The drawing under review shows one solid part. Ordinate dimensions are in mm from its lowest x, y, z. A direction names the side the tool comes from. Round coordinates to 2 decimals unless told otherwise and drop trailing zeros. Write each loop counter-clockwise with the first axis right and the second up, starting at its lowest first coordinate (ties: lowest second). Pieces come first, ordered by that corner, then holes. Notation, with made-up numbers: M 68.25,36.5 L 95.25,36.5 A17 cw 95.25,52.5 Z; hole C 74.25,16.25 d7. An arc over 180 degrees is marked long. Write item = value, one per line. Start each with the question number.
Item 1: Take a section at A-A, the plane y = 13. Give the boundary of the cut face in (x, z).
Item 2: To check wall thickness, follow line 1 along Z through (x, y) = (103.5, 17.75); line 2 along Z through (x, y) = (57.5, 19.75); line 3 along Z through (x, y) = (77, 12.5). State the ranges of each line that lie inside material, in increasing order.
Item 3: Take a section at D-D, the plane x = 87. Give the boundary of the cut face in (y, z), plus the area to 3 significant figures.
Item 4: Take a section at B-B, the plane x = 28. Give the boundary of the cut face in (y, z).
Item 5: For pin 1 Ø3 at (x, y) = (99.5, 6.5) entering from +Z; pin 2 Ø1.2 at (x, z) = (68, 95) entering from -Y; pin 3 Ø10 at (y, z) = (14, 183) entering from +X, all flat-tipped, find the tip position at first contact; note any pin that passes through.
Item 6: Take a section at C-C, the plane z = 54.5. Give the boundary of the cut face in (x, y).
Item 7: Tool access review of the marked faces 1, 2 and 3: name each direction out of +Z, -Z, +X, -X, +Y, -Y from which nothing blocks a thin tool from reaching the whole face with its end or side.
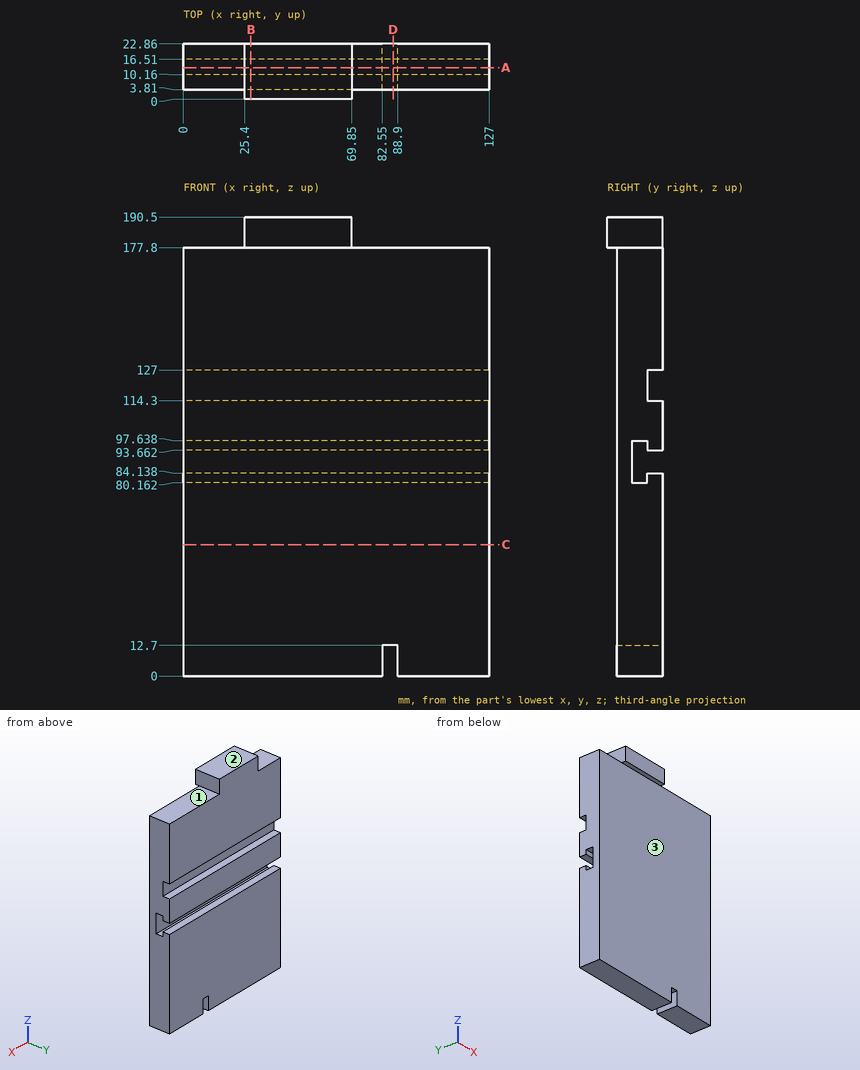
Response values:
q1.outline = M 0,0 L 82.55,0 L 82.55,12.7 L 88.9,12.7 L 88.9,0 L 127,0 L 127,80.16 L 0,80.16 Z; M 0,97.64 L 127,97.64 L 127,177.8 L 69.85,177.8 L 69.85,190.5 L 25.4,190.5 L 25.4,177.8 L 0,177.8 Z
q2.line_1 = 0 to 84.14, 93.66 to 114.3, 127 to 177.8
q2.line_2 = 0 to 84.14, 93.66 to 114.3, 127 to 190.5
q2.line_3 = 0 to 80.16, 97.64 to 177.8
q3.outline = M 3.81,12.7 L 22.86,12.7 L 22.86,84.14 L 16.51,84.14 L 16.51,80.16 L 10.16,80.16 L 10.16,97.64 L 16.51,97.64 L 16.51,93.66 L 22.86,93.66 L 22.86,114.3 L 16.51,114.3 L 16.51,127 L 22.86,127 L 22.86,177.8 L 3.81,177.8 Z
q3.area = 2,890 mm2
q4.outline = M 0,177.8 L 3.81,177.8 L 3.81,0 L 22.86,0 L 22.86,84.14 L 16.51,84.14 L 16.51,80.16 L 10.16,80.16 L 10.16,97.64 L 16.51,97.64 L 16.51,93.66 L 22.86,93.66 L 22.86,114.3 L 16.51,114.3 L 16.51,127 L 22.86,127 L 22.86,190.5 L 0,190.5 Z
q5.pin_1 = 177.8
q5.pin_2 = 3.81
q5.pin_3 = 69.85
q6.outline = M 0,3.81 L 127,3.81 L 127,22.86 L 0,22.86 Z
q7.face_1 = +Z, +X, +Y, -Y
q7.face_2 = +Z, +X, -X, +Y, -Y
q7.face_3 = -Z, +X, -X, -Y
